Autodesk Inventor part; units mm, degrees
ref_plane "XZ Plane" through (0, 0, 0) normal (0, 1, 0) x (-1, 0, 0)
sketch "Sketch1" plane through (0, 0, 0) normal (0, 1, 0) x (-1, 0, 0)
  line L0 (11.43, 15.875) -> (-11.43, 15.875)
  line L1 (-11.43, 15.875) -> (-11.43, -15.875)
  line L2 (-11.43, -15.875) -> (11.43, -15.875)
  line L3 (11.43, -15.875) -> (11.43, 15.875)
  line L4 (11.43, 15.875) -> (-11.43, -15.875) construction
  line L5 (-11.43, 15.875) -> (11.43, -15.875) construction
  point P0 (0, 0)
  dimension "d0" = 22.86
  dimension "d1" = 31.75
extrude "Extrusion1" add sketch "Sketch1" along normal blind 1.7272
sketch "Sketch2" plane through (0, 1.7272, 0) normal (0, 1, 0) x (1, 0, 0)
  line L0 (-11.2735, -13.081) -> (11.43, -13.081) construction
  line L1 (11.43, -15.875) -> (11.43, 15.875) construction
  circle A0 centre (-8.89, -13.081) radius 1.1684
  circle A1 centre (8.89, -13.081) radius 1.1684
  line L2 (-11.43, -15.875) -> (11.43, -15.875)
  line L3 (-11.43, 15.875) -> (-11.43, -15.875)
  point P0 (0, 0)
  dimension "d4" = 2.794
  dimension "d5" = 2.54
  dimension "d6" = 2.54
  dimension "d7" = 2.3368
  dimension "d8" = 2.3368
extrude "Extrusion2" cut sketch "Sketch2" against normal through all
equation "\"d0\" = boardWidth"
equation "\"d1\" = boardLength"
equation "\"d2\" = boardThickness"
equation "\"d4\" = centerLineForHoles"
equation "\"d5\" = holeDistanceFromEdge"
equation "\"d6\" = holeDistanceFromEdge"
equation "\"d7\" = holeDiam"
equation "\"d8\" = holeDiam"
equation "\"d9\" = boardThickness"
equation "\"boardWidth\" = 22.86"
equation "\"boardLength\" = 31.75"
equation "\"boardThickness\" = 1.7272"
equation "\"componentHeightAboveBoard\" = 3.9878"
equation "\"headerHeightAboveBard\" = 8.7376"
equation "\"holeDiam\" = 2.3368"
equation "\"centerLineForHoles\" = 2.794"
equation "\"holeDistanceFromEdge\" = 2.54"
equation "\"supportWidth\" = 25.4"
properties part number "ADXL_345" material "ABS Plastic"
Could you check a few things on this model? Use its own coordinates, in mm. Coordinates: 2 decimals unless noted, no trailing zeros. Loops run counter-clockwise (first coordinate to the right, second up) from the corner with the lowest first, then second, coordinate; pieces in that order, holes last.
1) Thinking about a two-plate mould opening in Z: for faces 1 (the face through (0, 1, -15.875)), 2 (the face through (-8.262, 0.876, 12.096)), 3 (the face through (0, 1, 15.875)), which applies, released by +Z, released by -Z, zero draft, split by the parting line, or undercut?
Reported:
face 1: released by -Z
face 2: undercut
face 3: released by +Z
2) Will this pin go through, and if not, where does the flat tip stop? pin 1 Ø2 at (x, z) = (-8.89, 13.081) entering from -Y.
Reported:
pin 1: passes through
3) Please list where this line runs through material, in increasing order: line 1 along Z through (x, y) = (-8.89, 0.8) (3 decimals).
Reported:
line 1: z = -15.875 to 11.913, 14.249 to 15.875
4) Imagine slicing it at A-A (x = 8.89). List the corners of the cut face in (y, z) for me (3 decimals).
Reported:
outline: (0, -15.875) - (1.727, -15.875) - (1.727, 11.913) - (0, 11.913) - close; (0, 14.249) - (1.727, 14.249) - (1.727, 15.875) - (0, 15.875) - close
